Check sheet for the modelled part. Datum: model origin and axes. Units: mm. A direction names the side the tool comes from. Round coordinates to 2 decimals unless told otherwise and drop trailing zeros. Loops run counter-clockwise (first coordinate to the right, second up) from the corner with the lowest first, then second, coordinate; pieces in that order, holes last. Notation, with made-up numbers: (81.25, 81.5) - (116.25, 81.5) arc R16 ccw to (116.25, 87.5) - close; hole circle Ø2 at (-25, 18). An arc over 180 degrees is marked (long way). Answer in a Markdown table with one row per item. Add a question column.
(1) Gauge pin test, flat ends, axial feed: pin 1 (6.5 mm diameter, centred on y = 28, z = -76, fed in from +X); pin 2 (8 mm diameter, centred on x = 2, y = 36, fed in from +Z); pin 3 (7.5 mm diameter, centred on x = 8.5, y = 45.5, fed in from -Z). Record the tip position at first contact, or that the pin passes through.
(2) Thickness scan on line 1 along Z through (x, y) = (5.5, 46.5); line 2 along Y through (x, z) = (11.75, -77.5); line 3 along Y through (x, z) = (12, -136). Record the ranges inside material, lowest first.
(3) Cross-section at B-B on y = 47.5. Enter the section's corners in (x, z), then the cut area to 3 significant figures.
(4) Mould release check, pull along Z, two halves, no side actions. Record for faces 1 (the flat face through (7, 15, -292.5)), 2 (the flat face through (7, 30, 234)), 3 (the flat face through (7, 30, 95)): +Z half, -Z half, draft (parallel to the pull), parting line (faces both ways), or undercut.
(5) Cross-section at C-C on z = 152.5. Enter the section's corners in (x, y).
(6) Cross-section at A-A on x = 11.75. Enter the section's corners in (y, z).
(7) Access from +Z, -Z, +X, -X, +Y, -Y to the whole of each face (thin tool, end or side, straight path). Record for faces 4 (the flat face through (7, 53, 152)), 5 (the flat face through (7, 30, -199)), 6 (the cylindrical face through (11.55, 23.81, -68.77)), 7 (the flat face through (15, 21, 4)), 8 (the flat face through (7, 41, 12.5)).
(8) Cross-section at D-D on z = 77.5. Enter the section's corners in (x, y).
from build123d import *

# Parameters (mm, degrees)
SALIENTE_EXTRUIR1_DEPTH = 15
CROQUIS2_R              = 11
CORTAR_EXTRUIR1_DEPTH   = 7


with BuildPart() as part:
    # Croquis1 → Saliente-Extruir1 (new body)
    with BuildSketch(Plane(origin=(0, 0, 0), x_dir=(0, 0, -1), z_dir=(1, 0, 0))):
        Polygon((-292.5, 0), (292.5, 0), (292.5, 30), (102.5, 30), (102.5, 53), (52.5, 53), (52.5, 30), (-12.5, 30), (-12.5, 53), (-62.5, 53), (-62.5, 30), (-127.5, 30), (-127.5, 53), (-177.5, 53), (-177.5, 30), (-292.5, 30), align=None)
    extrude(amount=SALIENTE_EXTRUIR1_DEPTH)

    # Croquis2 → Cortar-Extruir1 (cut)
    with BuildSketch(Plane(origin=(15, 0, 0), x_dir=(0, 0, -1), z_dir=(1, 0, 0))):
        with Locations((-37.5, 30.5)):
            Circle(CROQUIS2_R)
        with Locations((-152.5, 30.5)):
            Circle(CROQUIS2_R)
        with Locations((77.5, 30.5)):
            Circle(CROQUIS2_R)
    extrude(amount=-CORTAR_EXTRUIR1_DEPTH, mode=Mode.SUBTRACT)


solid = part.part
Answers:
| question | item | result |
|---|---|---|
| 1 | pin 1 | stops at x = 8 |
| 1 | pin 2 | stops at z = 177.5 |
| 1 | pin 3 | stops at z = -102.5 |
| 2 | line 1 | z = -102.5 to -52.5, 12.5 to 62.5, 127.5 to 177.5 |
| 2 | line 2 | y = 0 to 19.5, 41.5 to 53 |
| 2 | line 3 | y = 0 to 30 |
| 3 | outline | (0, -102.5) - (15, -102.5) - (15, -52.5) - (0, -52.5) - close; (0, 12.5) - (15, 12.5) - (15, 62.5) - (0, 62.5) - close; (0, 127.5) - (15, 127.5) - (15, 177.5) - (0, 177.5) - close |
| 3 | area | 2,250 mm^2 |
| 4 | face 1 | -Z half |
| 4 | face 2 | draft |
| 4 | face 3 | undercut |
| 5 | outline | (0, 0) - (15, 0) - (15, 19.5) - (8, 19.5) - (8, 41.5) - (15, 41.5) - (15, 53) - (0, 53) - close |
| 6 | outline | (0, -292.5) - (30, -292.5) - (30, -102.5) - (53, -102.5) - (53, -52.5) - (30, -52.5) - (30, 12.5) - (53, 12.5) - (53, 62.5) - (30, 62.5) - (30, 127.5) - (53, 127.5) - (53, 177.5) - (30, 177.5) - (30, 292.5) - (0, 292.5) - close; hole circle Ø22 at (30.5, -77.5); hole circle Ø22 at (30.5, 37.5); hole circle Ø22 at (30.5, 152.5) |
| 7 | face 4 | +Z, -Z, +X, -X, +Y |
| 7 | face 5 | -Z, +X, -X, +Y |
| 7 | face 6 | +X |
| 7 | face 7 | +Z, -Z, +X, +Y, -Y |
| 7 | face 8 | +X, -X, +Y |
| 8 | outline | (0, 0) - (15, 0) - (15, 30) - (0, 30) - close |
